Input: part model. Units: mm. Frame: model coordinates. A direction names the side the tool comes from. Coordinates: 2 decimals unless noted, no trailing zeros. Write each loop counter-clockwise with the first axis right and the second up, starting at its lowest first coordinate (ties: lowest second). Pieces come first, ordered by that corner, then holes. Notation, with made-up numbers: (-21.5, 5.25) - (-8.5, 5.25) arc R22 cw to (-8.5, 33.25) - close; hole circle Ø10 at (59, 79.25). An arc over 180 degrees is marked (long way). Use a Markdown table: item, result. Add a question column.
Q1. Material intervals for probe 1 along Y at (x, z) = (0, -6); probe 2 along Y at (x, z) = (0, -1); probe 3 along Z at (x, y) = (11.5, 18), sorted ascending. Write a range as from..to.
Q2. Section query C-C (z = 12). Return the cut outline in (x, y), then the cut area to 3 significant figures.
Q3. Set-up query: faces 1 (the face through (-0.07, -11.62, -4.02)), 2 (the face through (23.846, -7.509, 17.255)). Return all of +Z, -Z, +X, -X, +Y, -Y with unobstructed straight access to the full face (end or side cutting, diameter ignored); none if empty.
Q4. Section query A-A (z = 36.5). Return the cut outline in (x, y).
Q5. Mould query, pull axis Z, two halves, no side actions, for faces 3 (the face through (0, 2.5, 64)), 4 (the face through (0, 0, -5)), 5 (the face through (8.393, -0.211, -4.017)). Classes: released by +Z, released by -Z, zero draft, split by the parting line, or undercut.
Q6. Pin query (flat end, axial travel): P1, Ø3.5, axis at x = -10, y = 0, coming from the +Z side; P2, Ø6.5, axis at x = -1, y = -1, coming from the -Z side; P3, Ø1.5, axis at x = -0.5, z = 64.5, coming from the +Y side; P4, Ø6, axis at x = -20, z = 31.5, coming from the -Y side. Return the tip coordinate at first contact, or that it passes through.
Q7. Section query B-B (z = 64). Return the cut outline in (x, y), then the cut area to 3 significant figures.
Autodesk Inventor part; units mm, degrees
ref_plane "作業平面1" through (0, 0, -5) normal (0, 0, -1) x (-1, 0, 0)
ref_plane "作業平面2" through (0, 0, 68.5) normal (0, 0, 1) x (1, 0, 0)
ref_plane "YZ Plane" through (0, 0, 0) normal (1, 0, 0) x (0, 1, 0)
sketch "スケッチ1" plane through (0, 0, 0) normal (0, 0, 1) x (1, 0, 0)
  circle A0 centre (0, 0) radius 25
  dimension "d0" = 50
extrude "押し出し1" add sketch "スケッチ1" against normal blind 10
fillet "フィレット1" radius 4 1 edges at (-25, 0, -10)
sketch "スケッチ2" plane through (0, 0, 0) normal (0, 0, 1) x (1, 0, 0)
  circle A0 centre (0, 0) radius 25
  circle A1 centre (0, 0) radius 25
extrude "押し出し2" add sketch "スケッチ2" along normal blind 35
sketch "スケッチ3" plane through (0, 0, 0) normal (0, 0, 1) x (1, 0, 0)
  circle A0 centre (0, 0) radius 25
  circle A1 centre (0, 0) radius 25
  circle A2 centre (0, 0) radius 24.99
  dimension "d6" = 0.01
extrude "押し出し3" cut sketch "スケッチ3" against normal blind 0.01
sketch "スケッチ4" plane through (0, 0, -10) normal (0, 0, -1) x (-1, 0, 0)
  point P0 (0, 0)
  point P1 (0, 0)
hole "穴1" at (0, 0, -10) direction (0, 0, 1) diameter 8 end through all
sketch "スケッチ5" plane through (0, 0, -10) normal (0, 0, -1) x (-1, 0, 0)
  point P0 (0, 0)
  point P1 (0, -10)
  point P2 (10, 0)
  point P3 (0, 10)
  point P4 (-10, 0)
  dimension "d18" = 360
  dimension "d20" = 20
hole "穴2" at (0, -10, -10) at (-10, 0, -10) at (0, 10, -10) at (10, 0, -10) direction (0, 0, 1) diameter 3.242 depth 11.8 tip angle 118
ref_plane "作業平面1" through (0, 0, -5) normal (0, 0, -1) x (-1, 0, 0)
sketch "スケッチ6" plane through (0, 0, -5) normal (0, 0, -1) x (-1, 0, 0)
  circle A0 centre (0, 0) radius 4
  circle A1 centre (0, 0) radius 4
  dimension "d29" = 8
extrude "押し出し4" add sketch "スケッチ6" against normal blind 78.5
ref_plane "作業平面2" through (0, 0, 68.5) normal (0, 0, 1) x (1, 0, 0)
sketch "スケッチ7" plane through (0, 0, 68.5) normal (0, 0, 1) x (1, 0, 0)
  line L0 (-1.5, 4) -> (1.5, 4)
  line L1 (1.5, 4) -> (1.5, 2.5)
  line L2 (1.5, 2.5) -> (-1.5, 2.5)
  line L3 (-1.5, 2.5) -> (-1.5, 4)
  circle A0 centre (0, 0) radius 4
  point P0 (0, 2.5)
  dimension "d33" = 3
  dimension "d34" = 1.5
extrude "押し出し5" cut sketch "スケッチ7" against normal blind 10 contours L0 A0 L3 | L0 L1 A0 | A0 L1 L2 L3 picked at (0, 3)
properties part number "Rotator_N5065"
Values follow:
| question | item | result |
|---|---|---|
| 1 | probe 1 | -25..-11.62, -8.38..-4, 4..8.38, 11.62..25 |
| 1 | probe 2 | -25..-11.62, -8.38..8.38, 11.62..25 |
| 1 | probe 3 | -9.98..35 |
| 2 | outline | circle Ø50 at (0, 0) |
| 2 | area | 1,960 mm2 |
| 3 | face 1 | -Z |
| 3 | face 2 | +Z, -Z |
| 4 | outline | circle Ø8 at (0, 0) |
| 5 | face 3 | undercut |
| 5 | face 4 | released by -Z |
| 5 | face 5 | zero draft |
| 6 | P1 | z = 35 |
| 6 | P2 | z = -10 |
| 6 | P3 | y = 2.5 |
| 6 | P4 | y = -18.33 |
| 7 | outline | (-1.5, 2.5) - (-1.5, 3.71) arc R4 ccw (long way) to (1.5, 3.71) - (1.5, 2.5) - close |
| 7 | area | 46.1 mm2 |
